from build123d import *

# Parameters (mm, degrees)
F0_W     = 60
F0_H     = 75
F1_DEPTH = 0.5
F2_W     = 1
F2_H     = 75
F3_DEPTH = 45
F4_W     = 8
F4_H     = 75
F5_DEPTH = 0.5
F6_W     = 12.5
F6_H     = 12.5
F7_DEPTH = 0.5


with BuildPart() as f1:
    # F0 (on Top) → F1 (new body)
    with BuildSketch(Plane.XY):
        with Locations((1.917277, -3.667414)):
            Rectangle(F0_W, F0_H)
    extrude(amount=F1_DEPTH)

    # F2 (on face) → F3 (join)
    with BuildSketch(Plane.XY.offset(0.5)):
        with Locations((-27.582723, -3.667414)):
            Rectangle(F2_W, F2_H)
        with Locations((31.417277, -3.667414)):
            Rectangle(F2_W, F2_H)
    extrude(amount=F3_DEPTH)

    # F4 (on face) → F5 (join)
    with BuildSketch(Plane.XY.offset(45.5)):
        with Locations((-24.082723, -3.667414)):
            Rectangle(F4_W, F4_H)
        with Locations((27.917277, -3.667414)):
            Rectangle(F4_W, F4_H)
    extrude(amount=F5_DEPTH)

    # F6 (on face) → F7 (cut, through all)
    with BuildSketch(Plane(origin=(0, 0, 0), x_dir=(1, 0, 0), z_dir=(0, 0, -1))):
        with Locations((1.917277, 34.917414)):
            Rectangle(F6_W, F6_H)
    extrude(amount=-F7_DEPTH, mode=Mode.SUBTRACT)


solid = f1.part
Source: CAD feature listing. Evaluate the final solid. Frame: model axes, mm. A direction names the side the tool comes from. Give positions to 0.01 mm unless a question says otherwise; leave off trailing zeros. Write each loop counter-clockwise with the first axis right and the second up, starting at its lowest first coordinate (ties: lowest second). Pieces come first, ordered by that corner, then holes. Notation, with made-up numbers: (67.5, 9) -> (102.5, 9) arc R16 ccw to (102.5, 18) -> close; hole circle Ø7 at (29, 21). An arc over 180 degrees is marked (long way). Return JSON: item names as keys, results as strings. Group by question number.
1. Pin query (flat end, axial travel): pin 1 Ø17.5 at (x, y) = (-1, -4) entering from +Z. Return the tip coordinate at first contact, or that it passes through.
2. Section B-B, the plane x = -21. Output: boundary loops of the cut face in (y, z).
3. Access query for faces 1 (the face through (31.4, -41.167, 22.9)), 2 (the face through (-24, -3, 45.5)). Directions: +Z, -Z, +X, -X, +Y, -Y. A direction counts if a zero-diameter tool reaches every point of the face in a straight line with its end or side. Return the directions, or none.
4. Section C-C, the plane y = 19.5. Output: boundary loops of the cut face in (x, z).
5. Mould query, pull axis Z, two halves, no side actions, for faces 3 (the face through (27, -3, 45.5)), 4 (the face through (28, -3, 46)), 5 (the face through (31.917, -4, 23)), 6 (the face through (1, -3, 0)). Classes: +Z half, -Z half, draft (parallel to the pull), parting line (faces both ways), or undercut.
6. Material intervals for line 1 (X direction, y = -14, z = 29); line 2 (Z direction, x = 28.5, y = 20); line 3 (Z direction, x = -13.5, y = -16.5), sorted ascending. Write a range as from..to.
7. Section A-A, the plane z = 3. Output: boundary loops of the cut face in (x, y).
8. Section D-D, the plane x = 1. Output: boundary loops of the cut face in (y, z).
Determined:
{
 "1": {"pin 1": "stops at z = 0.5"},
 "2": {"outline": "(-41.17, 0) -> (33.83, 0) -> (33.83, 0.5) -> (-41.17, 0.5) -> close; (-41.17, 45.5) -> (33.83, 45.5) -> (33.83, 46) -> (-41.17, 46) -> close"},
 "3": {"face 1": "+Z, -Z, +X, -X, -Y", "face 2": "+Y, -Y"},
 "4": {"outline": "(-28.08, 0) -> (31.92, 0) -> (31.92, 46) -> (23.92, 46) -> (23.92, 45.5) -> (30.92, 45.5) -> (30.92, 0.5) -> (-27.08, 0.5) -> (-27.08, 45.5) -> (-20.08, 45.5) -> (-20.08, 46) -> (-28.08, 46) -> close"},
 "5": {"face 3": "undercut", "face 4": "+Z half", "face 5": "draft", "face 6": "-Z half"},
 "6": {"line 1": "x = -28.08..-27.08, 30.92..31.92", "line 2": "z = 0..0.5, 45.5..46", "line 3": "z = 0..0.5"},
 "7": {"outline": "(-28.08, -41.17) -> (-27.08, -41.17) -> (-27.08, 33.83) -> (-28.08, 33.83) -> close; (30.92, -41.17) -> (31.92, -41.17) -> (31.92, 33.83) -> (30.92, 33.83) -> close"},
 "8": {"outline": "(-28.67, 0) -> (33.83, 0) -> (33.83, 0.5) -> (-28.67, 0.5) -> close"}
}
